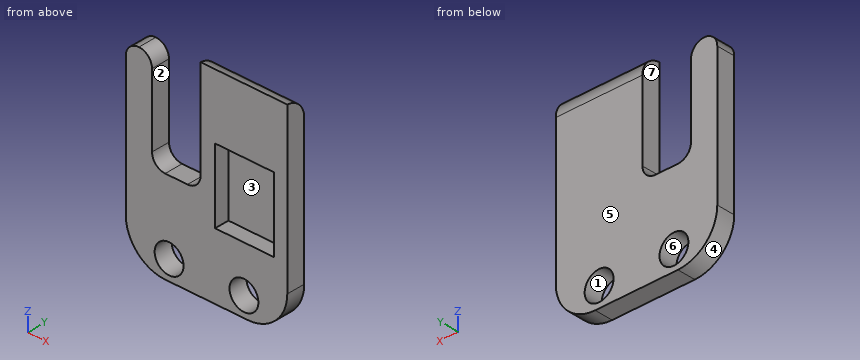
from build123d import *

# Parameters (mm, degrees)
BOSS_EXTRUDE1_DEPTH = 2.8
SKETCH4_R           = 2.2
CUT_EXTRUDE3_DEPTH  = 6
FILLET1_R           = 6
FILLET2_START       = -1
FILLET2_DEPTH       = 5
FILLET2_2_DEPTH     = 2.8
CUT_EXTRUDE7_START  = -2.8
SKETCH7_W           = 9
SKETCH7_H           = 11.2
CUT_EXTRUDE7_DEPTH  = 2.2
FILLET5_R           = 3


with BuildPart() as part:
    # Sketch1 → Boss-Extrude1 (new body)
    with BuildSketch(Plane(origin=(0, 0, 0), x_dir=(1, 0, 0), z_dir=(0, 1, 0))):
        Polygon((-16.635707691, 6.623874564), (7.964292309, 6.623874564), (7.964292309, -24.376125436), (-5.235707691, -24.376125436), (-5.235707691, -7.376125436), (-12.635707691, -7.376125436), (-12.635707691, -22.376125436), (-16.635707691, -22.376125436), align=None)
    extrude(amount=BOSS_EXTRUDE1_DEPTH)

    # Sketch4 → Cut-Extrude3 (cut)
    with BuildSketch(Plane(origin=(0, 2.8, 0), x_dir=(1, 0, 0), z_dir=(0, 1, 0))):
        with Locations(Location((-10.035707691, 3.623874564, 0), (0, 0, 270))):
            Circle(SKETCH4_R)
        with Locations(Location((1.364292309, 3.623874564, 0), (0, 0, 270))):
            Circle(SKETCH4_R)
    extrude(amount=-CUT_EXTRUDE3_DEPTH, mode=Mode.SUBTRACT)

    # Fillet1
    fillet1_edges = [part.edges().sort_by_distance(p)[0] for p in [
        (-16.635707691, 1.4, -6.623874564),
        (7.964292309, 1.4, -6.623874564),
    ]]
    fillet(fillet1_edges, radius=FILLET1_R)

    # Fillet2: read off the stored shape, not the designer's step
    # Fillet2 outline → Fillet2 (cut)
    with BuildSketch(Plane(origin=(0, 0, 0), x_dir=(1, 0, 0), z_dir=(0, 1, 0)).offset(FILLET2_START)):
        with BuildLine():
            Line((-16.635707691, -22.376125436), (-14.635707691, -22.376125436))
            ThreePointArc((-14.635707691, -22.376125436), (-16.049921254, -21.790338998), (-16.635707691, -20.376125436))
            Line((-16.635707691, -20.376125436), (-16.635707691, -22.376125436))
        make_face()
        with BuildLine():
            Line((-12.635707691, -22.376125436), (-12.635707691, -20.376125436))
            ThreePointArc((-12.635707691, -20.376125436), (-13.221494128, -21.790338999), (-14.635707691, -22.376125436))
            Line((-14.635707691, -22.376125436), (-12.635707691, -22.376125436))
        make_face()
    extrude(amount=FILLET2_DEPTH, mode=Mode.SUBTRACT)

    # Fillet2 2 outline → Fillet2 2 (add)
    with BuildSketch(Plane(origin=(0, 0, 0), x_dir=(1, 0, 0), z_dir=(0, 1, 0))):
        with BuildLine():
            ThreePointArc((-12.635707691, -9.376125436), (-12.049921253, -7.961911874), (-10.635707691, -7.376125436))
            Line((-10.635707691, -7.376125436), (-12.635707691, -7.376125436))
            Line((-12.635707691, -7.376125436), (-12.635707691, -9.376125436))
        make_face()
        with BuildLine():
            ThreePointArc((-7.235707691, -7.376125436), (-5.821494128, -7.961911874), (-5.235707691, -9.376125436))
            Line((-5.235707691, -9.376125436), (-5.235707691, -7.376125436))
            Line((-5.235707691, -7.376125436), (-7.235707691, -7.376125436))
        make_face()
    extrude(amount=FILLET2_2_DEPTH)

    # Sketch7 → Cut-Extrude7 (cut)
    with BuildSketch(Plane(origin=(0, 2.8, 0), x_dir=(1, 0, 0), z_dir=(0, 1, 0)).offset(CUT_EXTRUDE7_START)):
        with Locations((1.464292309, -8.976125436)):
            Rectangle(SKETCH7_W, SKETCH7_H)
    extrude(amount=CUT_EXTRUDE7_DEPTH, mode=Mode.SUBTRACT)

    # Fillet5
    # the kernel refuses this fillet: 3 mm, written as the material it takes off along each edge
    with BuildSketch(Plane(origin=(15.447607083, 2.8, 24.376125436), x_dir=(0, 0, -1), z_dir=(-1, 0, 0))) as fillet5_piece_1:
        with BuildLine():
            CenterArc((2.993325909, 3), FILLET5_R, 183.822553729, 86.177446271)
            Line((0, 2.8), (-0.059866518, 2.796))
            ThreePointArc((-0.059866518, 2.796), (-0.06, 1.4), (-0.06, 0))
            Line((-0.06, 0), (0, -0.06))
            Line((0, -0.06), (2.993325909, -0.06))
            Line((2.993325909, -0.06), (2.993325909, 0))
        make_face()
    extrude(amount=28.166629547, mode=Mode.SUBTRACT)


solid = part.part
Verification items for the finished model (mm, model axes). Face numbers are marked on the shaded views. A direction names the side the tool comes from. Coordinates: 2 decimals unless noted, no trailing zeros. Order: outer loops, then holes, each group sorted by start corner. A loop starts at its lowest first (then second) coordinate and runs counter-clockwise, first axis right, second up. Notation, with made-up numbers: (13, 30.25) -> (62, 30.25) arc R18 ccw to (62, 52.25) -> close; hole circle Ø3 at (-22.75, -2.5). An arc over 180 degrees is marked (long way). Use CSV: the item, a comma, the result in double quotes. Start each with the question number.
Q1. Section check A-A, the plane z = 18.5. Record the cut outline in (x, y).
Q2. Depth check by flat-ended pin: P1, Ø2.5, axis at x = -10.04, z = -3.62, coming from the -Y side; P2, Ø1.1, axis at x = 3.5, y = 1.5, coming from the +Z side; P3, Ø1.4, axis at x = -8.5, y = 2, coming from the +Z side; P4, Ø4.5, axis at x = 2, z = 6, coming from the -Y side. Enter the tip coordinate at first touch or a pass-through.
Q3. Section check D-D, the plane x = 4.75. Record the cut outline in (y, z).
Q4. Thickness scan on line 1 along X through (y, z) = (0.6, 13); line 2 along X through (y, z) = (0.95, 5); line 3 along X through (y, z) = (1.55, 17.5). Record the ranges inside material, lowest first.
Q5. Section check B-B, the plane x = -0.5. Record the cut outline in (y, z).
Q6. Draft check along X on the marked faces 4, 5, 6 and 7. Enter one of: +X half, -X half, draft (parallel to the pull), parting line (faces both ways), or undercut.
Q7. Section check C-C, the plane y = 1.85. Record the cut outline in (x, z), and give its area (3 significant figures).
Q8. Tool access check on the marked faces 1, 2 and 3. Record the directions out of +Z, -Z, +X, -X, +Y, -Y that give a thin tool (end or side, any length) a straight path to the whole face; none if there is none.
Returned:
1,outline,"(-16.64, 0) -> (-12.64, 0) -> (-12.64, 2.8) -> (-16.64, 2.8) -> close; (-5.24, 0) -> (7.96, 0) -> (7.96, 2.8) -> (-5.24, 2.8) -> close"
2,P1,"passes through"
2,P2,"stops at z = 24.15"
2,P3,"stops at z = 7.38"
2,P4,"stops at y = 2.2"
3,outline,"(0, -5.94) -> (2.8, -5.94) -> (2.8, 21.38) arc R3 ccw to (0, 24.38) -> (0, 14.58) -> (2.2, 14.58) -> (2.2, 3.38) -> (0, 3.38) -> close"
4,line 1,"x = -16.64 to -12.64, -5.24 to -3.04, 5.96 to 7.96"
4,line 2,"x = -16.64 to -3.04, 5.96 to 7.96"
4,line 3,"x = -16.64 to -12.64, -5.24 to 7.96"
5,outline,"(0, -6.62) -> (2.8, -6.62) -> (2.8, -4.79) -> (0, -4.79) -> close; (0, -2.46) -> (2.8, -2.46) -> (2.8, 21.38) arc R3 ccw to (0, 24.38) -> (0, 14.58) -> (2.2, 14.58) -> (2.2, 3.38) -> (0, 3.38) -> close"
6,face 4,"-X half"
6,face 5,"draft"
6,face 6,"undercut"
6,face 7,"undercut"
7,outline,"(-16.64, -0.62) arc R6 ccw to (-10.64, -6.62) -> (1.96, -6.62) arc R6 ccw to (7.96, -0.62) -> (7.96, 23.57) -> (-5.24, 23.57) -> (-5.24, 9.38) arc R2 cw to (-7.24, 7.38) -> (-10.64, 7.38) arc R2 cw to (-12.64, 9.38) -> (-12.64, 20.38) arc R2 ccw to (-16.64, 20.38) -> close; hole circle Ø4.4 at (-10.04, -3.62); hole (-3.04, 3.38) -> (5.96, 3.38) -> (5.96, 14.58) -> (-3.04, 14.58) -> close; hole circle Ø4.4 at (1.36, -3.62)"
7,area,"472 mm^2"
8,face 1,"+Y, -Y"
8,face 2,"+Z, +Y, -Y"
8,face 3,"-Y"
